For this review, take the finished solid that the model builds, in its own axes (mm). A direction names the side the tool comes from. Give positions to 0.01 mm unless a question says otherwise; leave off trailing zeros. Loops run counter-clockwise (first coordinate to the right, second up) from the corner with the lowest first, then second, coordinate; pieces in that order, holes last.
```python
from build123d import *

# Parameters (mm, degrees)
FILETE1_R     = 1.5
CHANFRO1_SIZE = 0.3


with BuildPart() as part:
    # Esboço1 → Revolução1 (revolve)
    with BuildSketch(Plane.XY, mode=Mode.PRIVATE) as revolu_o1_sk:
        Polygon((0, 0), (16.000553077, 0), (16, 0.5), (16, 3), (14, 3), (14, 2), (0, 2), align=None)
    revolve(revolu_o1_sk.sketch.rotate(Axis((0, 0, 0), (1, 0, 0)), 90), axis=Axis((0, 0, 0), (1, 0, 0)))

    # Filete1
    filete1_edges = [part.edges().sort_by_distance(p)[0] for p in [
        (16, 0, -3),
    ]]
    fillet(filete1_edges, radius=FILETE1_R)

    # Chanfro1
    chanfro1_edges = [part.edges().sort_by_distance(p)[0] for p in [
        (0, 0, -2),
    ]]
    chamfer(chanfro1_edges, length=CHANFRO1_SIZE)


solid = part.part
```
Item 1: For L1, parallel to Z at x = 3.25, y = -1.5; L2, parallel to Z at x = 11.25, y = -1.75; L3, parallel to X at y = 2.25, z = 1.25, list the stretches that pass through material, from the lowest coordinate up.
Answer:
L1: z = -1.32 to 1.32
L2: z = -0.97 to 0.97
L3: x = 14 to 15.55
Item 2: Clearance check with flat-ended pins moving along their axes: pin 1 Ø1.5 at (x, y) = (5, 1) entering from +Z; pin 2 Ø3 at (x, y) = (14, -2) entering from +Z; pin 3 Ø2 at (x, z) = (11.5, 0) entering from -Y. State where each tip first meets the part, or that it passes through.
Answer:
pin 1: stops at z = 1.98
pin 2: stops at z = 2.96
pin 3: stops at y = -2
Item 3: Tool access review of faces 1 (the cylindrical face through (7, 2, 0)), 2 (the flat face through (16, 0, -1)): name each direction out of +Z, -Z, +X, -X, +Y, -Y from which nothing blocks a thin tool from reaching the whole face with its end or side.
Answer:
face 1: -X
face 2: +Z, -Z, +X, +Y, -Y
Item 4: Take a section at A-A on x = 7. Give the boundary of the cut face in (y, z), and give its area (3 significant figures).
Answer:
outline: circle Ø4 at (0, 0)
area: 12.6 mm2
